Build history of the part. All positions in model axes, mm. A direction names the side the tool comes from. Round coordinates to 2 decimals unless told otherwise and drop trailing zeros. Loops run counter-clockwise (first coordinate to the right, second up) from the corner with the lowest first, then second, coordinate; pieces in that order, holes last. Notation, with made-up numbers: (-34.5, 65.25) - (22.5, 65.25) arc R29 cw to (22.5, 97.25) - close; hole circle Ø7 at (-22.5, 87). An arc over 180 degrees is marked (long way). Use one line per item in the form item = value. Start each with the question number.
Q1. Drill centre lines: line 1 (Y direction, x = 0, z = -3); line 2 (X direction, y = -8, z = 0); line 3 (X direction, y = 7, z = -2.2). Where is each one in solid material? Low to high.
Q2. Saw through at C-C (y = 8.75). Give the cut face in (x, z).
Q3. Saw through at A-A (y = -7). Give the cut face in (x, z).
Q4. Saw through at B-B (x = 0). Count the separate pieces of the cut face and the enclosed holes in it, then the cut area to 3 significant figures.
Q5. Pin check, flat tips, straight feed: pin 1 (5 mm diameter, centred on x = 0, y = -7, fed in from +Z); pin 2 (2.5 mm diameter, centred on x = 0, y = 7, fed in from +Z); pin 3 (1.5 mm diameter, centred on x = 0.5, z = 1.5, fed in from -Y). Stop position of each tip, or through.
Q6. Mould opens along Z. For faces 4 (the face through (1.72, 7.04, 4.16)), 5 (the face through (-1.5, 7.07, 2.72)), 6 (the face through (0.1, -5.1, 2.5)) say: released by +Z, released by -Z, zero draft, split by the parting line, or undercut.
Q7. 3-axis set-ups, long thin cutter, end or side, ignore diameter. For faces 1 (the face through (-2, 0, 0)), 2 (the face through (-1.11, 8.01, -2.78)), 3 (the face through (3.105, 0.042, 1.615)): which of +Z, -Z, +X, -X, +Y, -Y reach the whole face in a straight line?
```python
from build123d import *

# Parameters (mm, degrees)
SKETCH2_R               = 1.5
CUT_EXTRUDE1_DEPTH      = 21.988091862
SKETCH3_R               = 2.5
CUT_EXTRUDE2_DEPTH      = 10
CUT_EXTRUDE3_DEPTH      = 12.853269591
CUT_EXTRUDE3_DEPTH_BACK = 12.853269591
SKETCH4_R               = 1.5


with BuildPart() as part:
    # Sketch1 → Revolve1 (revolve)
    with BuildSketch(Plane.XY, mode=Mode.PRIVATE) as revolve1_sk:
        Polygon((3.5, -3), (3.5, 3), (4.5, 4), (4.5, 10), (0, 10), (0, -10), (4.5, -10), (4.5, -4), align=None)
    revolve(revolve1_sk.sketch.rotate(Axis((0, 10, 0), (0, -1, 0)), 90), axis=Axis((0, 10, 0), (0, -1, 0)))

    # Sketch2 → Cut-Extrude1 (cut, through all)
    with BuildSketch(Plane(origin=(0, 10, 0), x_dir=(1, 0, 0), z_dir=(0, 1, 0))):
        with Locations(Location((0, 0, 0), (0, 0, 270))):
            Circle(SKETCH2_R)
    extrude(amount=-CUT_EXTRUDE1_DEPTH, mode=Mode.SUBTRACT)

    # Sketch3 → Cut-Extrude2 (cut)
    with BuildSketch(Plane.XZ.offset(10)):
        with Locations(Location((0, 0, 0), (0, 0, 270))):
            Circle(SKETCH3_R)
    extrude(amount=-CUT_EXTRUDE2_DEPTH, mode=Mode.SUBTRACT)

    # Sketch4 → Cut-Extrude3 (cut, two sides: drawn at the far end of the back side and taken through both)
    with BuildSketch(Plane.XY.offset(-CUT_EXTRUDE3_DEPTH_BACK)):
        with Locations((0, 7)):
            Circle(SKETCH4_R)
        with Locations((0, -7)):
            Circle(SKETCH4_R)
    extrude(amount=CUT_EXTRUDE3_DEPTH + CUT_EXTRUDE3_DEPTH_BACK, mode=Mode.SUBTRACT)


solid = part.part
```
Report:
q1.line_1 = -10 to -8.5, -5.5 to 5.5, 8.5 to 10
q1.line_2 = -4.5 to -2.5, 2.5 to 4.5
q1.line_3 = -3.93 to -1.5, 1.5 to 3.93
q2.outline = circle Ø9 at (0, 0); hole circle Ø3 at (0, 0)
q3.outline = (-1.5, -4.24) - (-1.5, -2) arc R2.5 cw to (-1.5, 2) - (-1.5, 4.24) arc R4.5 ccw to start; (1.5, -4.24) arc R4.5 ccw to (1.5, 4.24) - (1.5, 2) arc R2.5 cw to (1.5, -2) - close
q4.separate_pieces = 6
q4.enclosed_holes = 0
q4.area = 56.0 mm²
q5.pin_1 = 4.5
q5.pin_2 = through
q5.pin_3 = 0
q6.face_4 = split by the parting line
q6.face_5 = zero draft
q6.face_6 = undercut
q7.face_1 = -Y
q7.face_2 = +Z, -Z
q7.face_3 = none
